Autodesk Inventor part; units mm, degrees
ref_plane "YZ Plane" through (0, 0, 0) normal (1, 0, 0) x (0, 1, 0)
ref_plane "XZ Plane" through (0, 0, 0) normal (0, 1, 0) x (-1, 0, 0)
ref_plane "XY Plane" through (0, 0, 0) normal (0, 0, 1) x (1, 0, 0)
sketch "Esboço1" plane through (0, 0, 0) normal (0, 1, 0) x (-1, 0, 0)
  line L0 (66, 0) -> (59, 0)
  line L1 (59, 0) -> (59, 2)
  line L2 (59, 2) -> (62, 2)
  line L3 (66, 2) -> (66, 0)
  line L4 (66, 0) -> (64, 0)
  line L5 (64, 4) -> (64, 7)
  line L6 (64, 7) -> (66, 7)
  line L7 (66, 7) -> (66, 0)
  arc A0 (62, 2) -> (64, 4) centre (62, 4) ccw
  point P0 (0, 0)
  dimension "d0" = 2
extrude "Extrusão1" add sketch "Esboço1" along normal blind 5
sketch "Esboço2" plane through (-59, 0, 0) normal (0, 0, -1) x (-1, 0, 0)
  circle A0 centre (2.5, 2.5) radius 1
  line L0 (0, 0) -> (7, 0)
  line L1 (0, 0) -> (0, 5)
  arc A1 (2.5, 5) -> (2.5, 0) centre (2.5, 2.5) ccw
  line L2 (3, 0) -> (0, 0)
  line L3 (3, 5) -> (0, 5)
  line L4 (2.5, 0) -> (0, 0)
  line L5 (0, 0) -> (0, 5)
  line L6 (0, 5) -> (2.5, 5)
  point P0 (-59, 0)
  point P1 (0, 2.5)
  dimension "d3" = 2
  dimension "d4" = 2.5
  dimension "d5" = 2.5
extrude "Extrusão2" cut sketch "Esboço2" against normal blind 4.25
sketch "Esboço3" plane through (-66, 0, 0) normal (-1, 0, 0) x (0, 0, 1)
  circle A0 centre (4.5, 2.5) radius 1
  line L0 (0, 5) -> (7, 5)
  line L1 (7, 0) -> (7, 5)
  arc A1 (4.5, 0) -> (4.5, 5) centre (4.5, 2.5) ccw
  line L2 (7, 0) -> (4, 0)
  line L3 (7, 5) -> (4, 5)
  line L4 (4.5, 0) -> (7, 0)
  line L5 (7, 0) -> (7, 5)
  line L6 (7, 5) -> (4.5, 5)
  point P0 (0, 0)
  point P1 (4.5, 5)
  point P2 (7, 2.5)
  dimension "d8" = 2.5
  dimension "d9" = 2.5
extrude "Extrusão3" cut sketch "Esboço3" against normal blind 4.25
sketch "Esboço4" plane through (-66, 0, 0) normal (0, 0, -1) x (-1, 0, 0)
  line L0 (0, -91.1) -> (0, 5)
  line L1 (-4.5, 0) -> (0, 0)
  line L2 (-4.5, 5) -> (0, 5)
  point P0 (-66, 0)
properties part number "conector 90°"
Geometry: final body of the model. Coordinates: model frame, mm. A direction names the side the tool comes from. Give positions to 0.01 mm unless a question says otherwise; leave off trailing zeros. Loops run counter-clockwise (first coordinate to the right, second up) from the corner with the lowest first, then second, coordinate; pieces in that order, holes last. Notation, with made-up numbers: M 5,78 L 41,78 A20 cw 41,103 Z; hole C -31,33.25 d6. An arc over 180 degrees is marked long. Put each result on its own line as item: value. Start each with the question number.
1) Cut plane D-D (z = 4.75). Output: boundary loops of the cut face in (x, y).
2) Cut plane A-A (y = 2.5). Output: boundary loops of the cut face in (x, z).
3) Access query for faces 1 (the flat face through (-60, 2, 2)), 2 (the flat face through (-63, 2, 0)). Directions: +Z, -Z, +X, -X, +Y, -Y. A direction counts if a zero-diameter tool reaches every point of the face in a straight line with its end or side. Return the directions, or none.
4) Pull-direction query (Y, two-part tool) for faces 3 (the flat face through (-64, 5, 2)), 4 (the flat face through (-66, 2, 3)), 5 (the cylindrical face through (-60.5, 2.5, 1)), 6 (the cylindrical face through (-65, 2.5, 3.5)); classes: pulls with the +Y half, pulls with the -Y half, needs draft (parallel to the pull), parting line crosses it, or undercut.
5) Contact query for flat-ended pins moving along their axis: pin 1 (1.5 mm diameter, centred on y = 3.5, z = 5, fed in from +X); pin 2 (2.5 mm diameter, centred on x = -60.5, y = 3, fed in from +Z). Output: stop coordinate, or through.
6) Cut plane C-C (z = 1). Output: boundary loops of the cut face in (x, y).
7) Ray query, line 1 along Z through (x, y) = (-64.45, 2.5); line 2 along Y through (x, z) = (-65.25, 4.5); line 3 along Z through (x, y) = (-60.25, 3.35). Return the intervals inside material, ascending.
8) Cut plane B-B (x = -61). Output: boundary loops of the cut face in (y, z), then the cut area to 3 significant figures.
Verdict:
1. outline: M -66,0.01 L -64,0.01 L -64,1.53 L -66,1.53 Z; M -66,3.47 L -64,3.47 L -64,4.99 L -66,4.99 Z
2. outline: M -66,0 L -62.5,0 L -62.5,2.06 A2 cw -63.94,3.5 L -66,3.5 Z; M -66,5.5 L -64,5.5 L -64,7 L -66,7 Z; M -60.5,0 L -59,0 L -59,2 L -60.5,2 Z
3. face 1: +Z, +X, +Y, -Y
3. face 2: -Z, +X, -X, +Y, -Y
4. face 3: pulls with the +Y half
4. face 4: needs draft
4. face 5: undercut
4. face 6: undercut
5. pin 1: x = -64
5. pin 2: z = 2
6. outline: M -66,0 L -61.5,0 A2.5 ccw -61.5,5 L -66,5 Z; hole C -61.5,2.5 d2
7. line 1: 0 to 3.5, 5.5 to 7
7. line 2: 0 to 1.5, 3.5 to 5
7. line 3: 0 to 2
8. outline: M 0.05,0 L 1.63,0 L 1.63,2 L 0.05,2 Z; M 3.37,0 L 4.95,0 L 4.95,2 L 3.37,2 Z
8. area: 6.33 mm2
